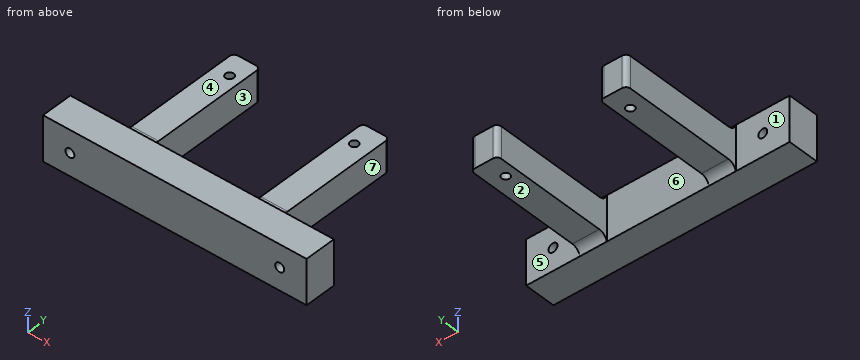
from build123d import *

# Parameters (mm, degrees)
SKETCH1_W         = 58.78
SKETCH1_H         = 10
BASE_DEPTH        = 7
SKETCH4_W         = 6
SKETCH4_H         = 35
SKETCH4_R         = 0.915
FLANGE_DEPTH      = 3.5
HOLE_R            = 1
BOTTOM_HOLE_DEPTH = 7
BOTTOM_FILLET_R   = 2
TOP_FILLET_R      = 1


with BuildPart() as part:
    # Sketch1 → Base (new body)
    with BuildSketch(Plane(origin=(0, 0, 0), x_dir=(1, 0, 0), z_dir=(0, 1, 0))):
        Rectangle(SKETCH1_W, SKETCH1_H)
    extrude(amount=BASE_DEPTH)

    # Sketch4 → Flange (add, symmetric)
    # profile 1 of 2: a face of its own
    with BuildSketch(Plane.XY):
        with Locations((-14.39, 17.5)):
            Rectangle(SKETCH4_W, SKETCH4_H)
        with Locations((-13.9, 30)):
            Circle(SKETCH4_R, mode=Mode.SUBTRACT)
    # profile 2 of 2: a face of its own
    with BuildSketch(Plane.XY):
        with Locations((14.39, 17.5)):
            Rectangle(SKETCH4_W, SKETCH4_H)
        with Locations((13.9, 30)):
            Circle(SKETCH4_R, mode=Mode.SUBTRACT)
    extrude(amount=FLANGE_DEPTH, both=True)

    # Hole → Bottom Hole (cut)
    with BuildSketch(Plane(origin=(0, 7, 0), x_dir=(1, 0, 0), z_dir=(0, 1, 0))):
        with Locations(Location((-23.39, 0, 0), (0, 0, 270))):
            Circle(HOLE_R)
        with Locations(Location((23.39, 0, 0), (0, 0, 270))):
            Circle(HOLE_R)
    extrude(amount=-BOTTOM_HOLE_DEPTH, mode=Mode.SUBTRACT)

    # Bottom Fillet
    # the kernel refuses this fillet: 2 mm, written as the material it adds along each edge
    with BuildSketch(Plane(origin=(-11.39, 7, -3.5), x_dir=(0, 0, -1), z_dir=(-1, 0, 0)), Plane(origin=(11.39, 7, 3.5), x_dir=(0, 0, 1), z_dir=(1, 0, 0))) as bottom_fillet_piece_1:
        with BuildLine():
            CenterArc((2, -1.936491673), BOTTOM_FILLET_R, 104.477512186, 75.522487814)
            Line((0, -1.936491673), (-0.04, -1.936491673))
            Line((-0.04, -1.936491673), (-0.04, 0))
            Line((-0.04, 0), (0, 0.04))
            ThreePointArc((0, 0.04), (0.75, 0.04), (1.49, 0.038729833))
            Line((1.49, 0.038729833), (1.5, 0))
        make_face()
    extrude(amount=6)
    with BuildSketch(Plane(origin=(-11.39, 7, 3.5), x_dir=(0, 0, 1), z_dir=(-1, 0, 0)), Plane(origin=(11.39, 7, -3.5), x_dir=(0, 0, -1), z_dir=(1, 0, 0))) as bottom_fillet_piece_2:
        with BuildLine():
            CenterArc((2, 1.936491673), BOTTOM_FILLET_R, 180, 75.522487814)
            Line((0, 1.936491673), (-0.04, 1.936491673))
            Line((-0.04, 1.936491673), (-0.04, 0))
            Line((-0.04, 0), (0, -0.04))
            ThreePointArc((0, -0.04), (0.75, -0.04), (1.49, -0.038729833))
            Line((1.49, -0.038729833), (1.5, 0))
        make_face()
    extrude(amount=6)

    # Top Fillet
    top_fillet_edges = [part.edges().sort_by_distance(p)[0] for p in [
        (-17.39, 35, 0),
        (-11.39, 35, 0),
        (11.39, 35, 0),
        (17.39, 35, 0),
    ]]
    fillet(top_fillet_edges, radius=TOP_FILLET_R)


solid = part.part
Could you check a few things on this model? Use its own coordinates, in mm. Face numbers are marked on the shaded views. A direction names the side the tool comes from. Round coordinates to 2 decimals unless told otherwise and drop trailing zeros. Order: outer loops, then holes, each group sorted by start corner. A loop starts at its lowest first (then second) coordinate and runs counter-clockwise, first axis right, second up.
Q1. Imagine slicing it at B-B, the plane y = 30. List the corners of the cut face in (x, z) for me (3 decimals), then the cut area to 3 significant figures.
Geometry says:
outline: (-17.39, -3.5) - (-14.815, -3.5) - (-14.815, 3.5) - (-17.39, 3.5) - close; (-12.985, -3.5) - (-11.39, -3.5) - (-11.39, 3.5) - (-12.985, 3.5) - close; (11.39, -3.5) - (12.985, -3.5) - (12.985, 3.5) - (11.39, 3.5) - close; (14.815, -3.5) - (17.39, -3.5) - (17.39, 3.5) - (14.815, 3.5) - close
area: 58.4 mm2
Q2. Imagine slicing it at D-D, the plane y = 24. List the corners of the cut face in (x, z) for me.
Geometry says:
outline: (-17.39, -3.5) - (-11.39, -3.5) - (-11.39, 3.5) - (-17.39, 3.5) - close; (11.39, -3.5) - (17.39, -3.5) - (17.39, 3.5) - (11.39, 3.5) - close
Q3. Imagine slicing it at C-C, the plane x = 23.39. List the corners of the cut face in (y, z) for me, then the cut area to 3 significant figures.
Geometry says:
outline: (0, -5) - (7, -5) - (7, -1) - (0, -1) - close; (0, 1) - (7, 1) - (7, 5) - (0, 5) - close
area: 56.0 mm2
Q4. Thinking about a two-plate mould opening in X: for the marked faces 5, 6 and 7, which applies, released by +X, released by -X, zero draft, split by the parting line, or undercut?
Geometry says:
face 5: zero draft
face 6: undercut
face 7: released by +X
Q5. Which directions (+Z, -Z, +X, -X, +Y, -Y) give clear straight access to the entire face, cutting with the end or side of a thin tool? Please do the marked faces 1, 2, 3 and 4.
Geometry says:
face 1: +Z, -Z, -X, +Y
face 2: -Z, +X, -X, +Y
face 3: +Z, -Z, +Y
face 4: +Z, +X, -X, +Y
Q6. Imagine slicing it at A-A, the plane z = 0. List the corners of the cut face in (x, y) for me (3 decimals), then the cut area to 3 significant figures.
Geometry says:
outline: (-29.39, 0) - (-24.39, 0) - (-24.39, 7) - (-29.39, 7) - close; (-22.39, 0) - (22.39, 0) - (22.39, 7) - (17.39, 7) - (17.39, 34) arc R1 ccw to (16.39, 35) - (12.39, 35) arc R1 ccw to (11.39, 34) - (11.39, 7) - (-11.39, 7) - (-11.39, 34) arc R1 ccw to (-12.39, 35) - (-16.39, 35) arc R1 ccw to (-17.39, 34) - (-17.39, 7) - (-22.39, 7) - close; (24.39, 0) - (29.39, 0) - (29.39, 7) - (24.39, 7) - close; hole circle Ø1.83 at (-13.9, 30); hole circle Ø1.83 at (13.9, 30)
area: 713 mm2
Q7. I'm going to push flat-ended pins straight in: P1, Ø5, axis at x = -15.5, y = 28, coming from the -Z side; P2, Ø5, axis at y = 23, z = 0.5, coming from the +X side; P3, Ø1, axis at x = -18, z = 0, coming from the +Y side; P4, Ø3, axis at x = -9, z = -3.5, coming from the -Y side. Where does each tip first touch, or does it pass through?
Geometry says:
P1: stops at z = -3.5
P2: stops at x = 17.39
P3: stops at y = 7
P4: stops at y = 0
Q8. Please list where these lines run through material, in increasing order: probe 1 along X at (y, z) = (4.75, 0); probe 2 along X at (y, z) = (26, 3); probe 3 along Y at (x, z) = (-13.9, -1) (3 decimals).
Geometry says:
probe 1: x = -29.39 to -24.39, -22.39 to 22.39, 24.39 to 29.39
probe 2: x = -17.39 to -11.39, 11.39 to 17.39
probe 3: y = 0 to 29.085, 30.915 to 35
